```python
from build123d import *

# Parameters (mm, degrees)
F0_W     = 238.125
F0_H     = 168.275
F1_DEPTH = 6.35
F2_R     = 5.08
F4_DEPTH = 25.4
F6_DEPTH = 25.4
F7_R     = 0.7874


with BuildPart() as f1:
    # F0 (on Top) → F1 (new body)
    with BuildSketch(Plane.XY):
        Rectangle(F0_W, F0_H)
    extrude(amount=F1_DEPTH)

    # F2
    f2_edges = [f1.edges().sort_by_distance(p)[0] for p in [
        (-119.0625, 84.1375, 3.175),
        (-119.0625, -84.1375, 3.175),
        (119.0625, 84.1375, 3.175),
        (119.0625, -84.1375, 3.175),
    ]]
    fillet(f2_edges, radius=F2_R)

    # F3 (on face) → F4 (cut)
    with BuildSketch(Plane.XY.offset(6.35)):
        Polygon((-63.021223, -5.113947), (53.750796, -55.181694), (95.367796, -38.174427), (77.802704, -30.800822), (95.204413, 10.652795), (53.750796, 28.054503), (61.124402, 45.619595), align=None)
    extrude(amount=-F4_DEPTH, mode=Mode.SUBTRACT)

    # F5 (on face) → F6 (cut)
    with BuildSketch(Plane.XY.offset(6.35)):
        Polygon((55.413376, 28.733936), (63.482172, 47.95508), (-66.309597, -5.085824), (53.739022, -56.558461), (98.686428, -38.190185), (79.465284, -30.121389), (96.866992, 11.332227), align=None)
    extrude(amount=-F6_DEPTH, mode=Mode.SUBTRACT)

    # F7
    f7_edges = [f1.edges().sort_by_distance(p)[0] for p in [
        (-66.309597, -5.085824, 3.175),
        (63.482172, 47.95508, 3.175),
        (96.866992, 11.332227, 3.175),
        (55.413376, 28.733936, 3.175),
        (79.465284, -30.121389, 3.175),
        (98.686428, -38.190185, 3.175),
        (53.739022, -56.558461, 3.175),
    ]]
    fillet(f7_edges, radius=F7_R)


solid = f1.part
```
For this review, take the finished solid that the model builds, in its own axes (mm). A direction names the side the tool comes from. Coordinates: 2 decimals unless noted, no trailing zeros. Loops run counter-clockwise (first coordinate to the right, second up) from the corner with the lowest first, then second, coordinate; pieces in that order, holes last.
1. Add section A-A, the plane y = 42.5. Give the boundary of the cut face in (x, z), then the cut area to 3 significant figures.
2. Add section C-C, the plane x = -61.5. Give the boundary of the cut face in (y, z).
3. Insertion check: P1, Ø2, axis at x = 57, y = 42.5, coming from the -Z side. The pin has a flat end and moves straight along its axis. Give the tip position at first contact, or say it passes through.
4. Add section B-B, the plane z = 5.25. Give the boundary of the cut face in (x, y).
5. Mouldability with a two-part tool opening along Y and no side actions: class faces 3 (the flat face through (76.42, 19.916, 3.219)), 4 (the cylindrical face through (117.614, 82.61, 3.219)), 5 (the flat face through (-2, -84.138, 3)) as +Y half, -Y half, draft (parallel to the pull), parting line (faces both ways), or undercut.
6. For faces 1 (the flat face through (88.7, -34, 3.2)), 2 (the flat face through (-28, 20, 6.35)), list the 3-axis set-ups (+Z, -Z, +X, -X, +Y, -Y) from which the entire face can be reached by the end or side of a thin tool; tool diameter is ignored.
7. For line 1 (Y direction, x = 86, z = 6); line 2 (Y direction, x = 94, z = 4.75); line 3 (Y direction, x = 97, z = 2.25), list the stretches that pass through material, from the lowest coordinate up.
Result:
1. outline: (-119.06, 0) - (50.13, 0) - (50.13, 6.35) - (-119.06, 6.35) - close; (61.19, 0) - (119.06, 0) - (119.06, 6.35) - (61.19, 6.35) - close
1. area: 1,440 mm2
2. outline: (-84.14, 0) - (-7.15, 0) - (-7.15, 6.35) - (-84.14, 6.35) - close; (-3.12, 0) - (84.14, 0) - (84.14, 6.35) - (-3.12, 6.35) - close
3. P1: passes through
4. outline: (-119.06, -79.06) arc R5.08 ccw to (-113.98, -84.14) - (113.98, -84.14) arc R5.08 ccw to (119.06, -79.06) - (119.06, 79.06) arc R5.08 ccw to (113.98, 84.14) - (-113.98, 84.14) arc R5.08 ccw to (-119.06, 79.06) - close; hole (-64.58, -5.83) - (53.44, -56.43) arc R0.79 ccw to (54.04, -56.43) - (96.93, -38.91) arc R0.79 ccw to (96.93, -37.45) - (80.19, -30.43) arc R0.79 cw to (79.77, -29.4) - (96.56, 10.61) arc R0.79 ccw to (96.14, 11.64) - (56.14, 28.43) arc R0.79 cw to (55.72, 29.46) - (62.75, 46.2) arc R0.79 ccw to (61.72, 47.24) - (-64.57, -4.37) arc R0.79 ccw to start
5. face 3: undercut
5. face 4: +Y half
5. face 5: -Y half
6. face 1: +Z, -Z
6. face 2: +Z, +X, -X, +Y, -Y
7. line 1: y = -84.14 to -43.37, -32.86 to -14.55, 15.89 to 84.14
7. line 2: y = -84.14 to -40.11, -36.22 to 4.5, 12.54 to 84.14
7. line 3: y = -84.14 to -38.87, -37.49 to 84.14
